Check sheet for the modelled part. Datum: model origin and axes. Units: mm. Give positions to 0.01 mm unless a question says otherwise; leave off trailing zeros. Write each loop counter-clockwise with the first axis right and the second up, starting at its lowest first coordinate (ties: lowest second). Pieces come first, ordered by that corner, then holes. Notation, with made-up numbers: (-15.75, 45) -> (39.25, 45) arc R27 cw to (39.25, 82) -> close; hole circle Ø8 at (10, 89). An arc over 180 degrees is marked (long way). Write each question's results on one line, items separated by ' | '. Start each with the question number.
```python
from build123d import *

# Parameters (mm, degrees)
CUT_EXTRUDE1_DEPTH = 1
CUT_EXTRUDE1_TAPER = 10


with BuildPart() as part:
    # Sketch2 → Revolve1 (revolve)
    with BuildSketch(Plane.XY):
        with BuildLine():
            Line((-2.425, 0), (-2.425, -12.7))
            Line((-2.425, -12.7), (-1.95, -12.7))
            Line((-1.95, -12.7), (-1.95, -17.05))
            Line((-1.95, -17.05), (0, -19))
            Line((0, -19), (0, 0))
            Line((0, 0), (0, 1.4))
            Line((0, 1.4), (-4.514142843, 1.4))
            ThreePointArc((-4.514142843, 1.4), (-4.8, 0.7), (-4.514142843, 0))
            Line((-4.514142843, 0), (-2.425, 0))
        make_face()
    revolve(axis=Axis((0, -19, 0), (0, -1, 0)))

    # Sketch3 → Cut-Extrude1 (cut)
    with BuildSketch(Plane(origin=(0, 1.4, 0), x_dir=(1, 0, 0), z_dir=(0, 1, 0))):
        Polygon((-0.45, 2), (-0.45, 0.45), (-2, 0.45), (-2, -0.45), (-0.45, -0.45), (-0.45, -2), (0.45, -2), (0.45, -0.45), (2, -0.45), (2, 0.45), (0.45, 0.45), (0.45, 2), align=None)
    extrude(amount=-CUT_EXTRUDE1_DEPTH, taper=CUT_EXTRUDE1_TAPER, mode=Mode.SUBTRACT)


solid = part.part
```
Item 1: Mould release check, pull along X, two halves, no side actions. Record for faces 1 (the conical face through (-1, -18, 0)), 2 (the flat face through (1, 1.4, 1)), 3 (the flat face through (0, 0.4, 0)): pulls with the +X half, pulls with the -X half, needs draft (parallel to the pull), parting line crosses it, or undercut.
Item 2: Thickness scan on probe 1 along Y at (x, z) = (-3, 2.25); probe 2 along Z at (x, y) = (-0.5, -17.75); probe 3 along Z at (x, y) = (1.75, -3.5). Record the ranges inside material, lowest first. Write a range as from..to.
Item 3: Section check A-A on y = -14.75. Record the boundary of the cut face in (x, z).
Item 4: Depth check by flat-ended pin: pin 1 Ø3 at (y, z) = (-13, 2.5) entering from -X; pin 2 Ø1.1 at (x, z) = (0, -0.5) entering from +Y; pin 3 Ø4 at (y, z) = (-10, 3.5) entering from -X; pin 4 Ø1.5 at (y, z) = (-12.5, -2.5) entering from -X. Enter the tip coordinate at first touch or a pass-through.
Item 5: Section check B-B on y = -2.75. Record the boundary of the cut face in (x, z) (3 decimals), then the cut area to 3 significant figures.
Check sheet entries:
1) face 1: parting line crosses it | face 2: needs draft | face 3: undercut
2) probe 1: y = 0..1.4 | probe 2: z = -1.15..1.15 | probe 3: z = -1.68..1.68
3) outline: circle Ø3.9 at (0, 0)
4) pin 1: stops at x = -2.2 | pin 2: stops at y = 1.4 | pin 3: stops at x = -1.91 | pin 4: stops at x = -1.68
5) outline: circle Ø4.85 at (0, 0) | area: 18.5 mm^2
